Input: part model. Units: mm. Frame: model coordinates. A direction names the side the tool comes from. Coordinates: 2 decimals unless noted, no trailing zeros. Loops run counter-clockwise (first coordinate to the right, second up) from the corner with the lowest first, then second, coordinate; pieces in that order, holes last. Notation, with made-up numbers: (43, -40) - (71, -40) arc R22 cw to (71, -20) - close; hole circle Ø9 at (42.25, -2.75). An arc over 180 degrees is marked (long way). Write item = value, one per line. Start each with the question number.
from build123d import *

# Parameters (mm, degrees)
SERVO_ROD_HOLDERS_W                 = 10.16
SERVO_ROD_HOLDERS_H                 = 25.4
SERVO_ROD_HOLDERS_W_2               = 7.62
BASE_OF_THE_HOLDERS_DEPTH           = 0.508
SERVO_ROD_HOLDERS_3_W               = 7.62
SERVO_ROD_HOLDERS_3_H               = 25.4
TWO_HOLDERS_EXTRUDE_DEPTH           = 25.908
SKETCH2_R                           = 5.08
PLACEMENT_FOR_ROD_EXTRUDE_CUT_DEPTH = 25.4
SERVO_ROD_HOLDERS_4_W               = 12.7
SERVO_ROD_HOLDERS_4_H               = 25.4
EXTENSION_FOR_SCREWS_DEPTH          = 0.508


with BuildPart() as part:
    # Servo Rod Holders → Base of the Holders (new body)
    with BuildSketch(Plane.XY):
        with Locations((3.091913881, 0.940064131)):
            Rectangle(SERVO_ROD_HOLDERS_W, SERVO_ROD_HOLDERS_H)
        with Locations((-5.798086119, 0.940064131)):
            Rectangle(SERVO_ROD_HOLDERS_W_2, SERVO_ROD_HOLDERS_H)
        with Locations((11.981913881, 0.940064131)):
            Rectangle(SERVO_ROD_HOLDERS_W_2, SERVO_ROD_HOLDERS_H)
    extrude(amount=BASE_OF_THE_HOLDERS_DEPTH)

    # Servo Rod Holders_3 → Two Holders Extrude (add)
    with BuildSketch(Plane.XY):
        with Locations((11.981913881, 0.940064131)):
            Rectangle(SERVO_ROD_HOLDERS_3_W, SERVO_ROD_HOLDERS_3_H)
        with Locations((-5.798086119, 0.940064131)):
            Rectangle(SERVO_ROD_HOLDERS_3_W, SERVO_ROD_HOLDERS_3_H)
    extrude(amount=TWO_HOLDERS_EXTRUDE_DEPTH)

    # Sketch2 → Placement for Rod Extrude Cut (cut)
    with BuildSketch(Plane(origin=(15.791913881, 0, 0), x_dir=(0, 0, -1), z_dir=(1, 0, 0))):
        with Locations((-15.24, 0.940064131)):
            Circle(SKETCH2_R)
    extrude(amount=-PLACEMENT_FOR_ROD_EXTRUDE_CUT_DEPTH, mode=Mode.SUBTRACT)

    # Servo Rod Holders_4 → Extension for Screws (add)
    with BuildSketch(Plane.XY):
        with Locations((-15.958086119, 0.940064131)):
            Rectangle(SERVO_ROD_HOLDERS_4_W, SERVO_ROD_HOLDERS_4_H)
        with Locations((22.141913881, 0.940064131)):
            Rectangle(SERVO_ROD_HOLDERS_4_W, SERVO_ROD_HOLDERS_4_H)
    extrude(amount=EXTENSION_FOR_SCREWS_DEPTH)


solid = part.part
Item 1: Cut plane D-D on y = -2.5. Return loops of the section in (x, z), plus the area to 3 significant figures.
Item 2: Access query for faces 1 (the flat face through (-3, 13.64, 13)), 2 (the flat face through (22, 1, 0.508)), 3 (the flat face through (3, 1, 0.508)). Directions: +Z, -Z, +X, -X, +Y, -Y. A direction counts if a zero-diameter tool reaches every point of the face in a straight line with its end or side. Return the directions, or none.
Item 3: Pin query (flat end, axial travel): pin 1 (1.5 mm diameter, centred on y = 0, z = 22.5, fed in from -X); pin 2 (2 mm diameter, centred on y = 4, z = 23.5, fed in from +X); pin 3 (6.5 mm diameter, centred on x = 23.5, y = 1, fed in from +Z). Return the tip coordinate at first contact, or that it passes through.
Item 4: Cut plane A-A on z = 3. Return loops of the section in (x, y).
Item 5: Pull-direction query (Z, two-part tool) for faces 4 (the flat face through (-9.608, -2, 10)), 5 (the cylindrical face through (12.035, 2.466, 10.395)), 6 (the cylindrical face through (-5.745, 2.466, 10.395)), 7 (the flat face through (-16, 1, 0.508)); classes: pulls with the +Z half, pulls with the -Z half, needs draft (parallel to the pull), parting line crosses it, or undercut.
Item 6: Cut plane C-C on y = 7.25. Return loops of the section in (x, z), plus the area to 3 significant figures.
Item 7: Cut plane B-B on z = 15.24. Return loops of the section in (x, y).
Item 8: Ray query, line 1 (X direction, y = -7.25, z = 21); line 2 (Z direction, x = -14, y = -4.5); line 3 (Y direction, x = -5.75, z = 15.24). Return the intervals inside material, ascending.
Recorded:
q1.outline = (-22.31, 0) - (28.49, 0) - (28.49, 0.51) - (15.79, 0.51) - (15.79, 11.5) - (8.17, 11.5) - (8.17, 0.51) - (-1.99, 0.51) - (-1.99, 11.5) - (-9.61, 11.5) - (-9.61, 0.51) - (-22.31, 0.51) - close; (-9.61, 18.98) - (-1.99, 18.98) - (-1.99, 25.91) - (-9.61, 25.91) - close; (8.17, 18.98) - (15.79, 18.98) - (15.79, 25.91) - (8.17, 25.91) - close
q1.area = 299 mm²
q2.face_1 = +Z, -Z, +X, -X, +Y
q2.face_2 = +Z, +X, +Y, -Y
q2.face_3 = +Z, +Y, -Y
q3.pin_1 = -9.61
q3.pin_2 = 15.79
q3.pin_3 = 0.51
q4.outline = (-9.61, -11.76) - (-1.99, -11.76) - (-1.99, 13.64) - (-9.61, 13.64) - close; (8.17, -11.76) - (15.79, -11.76) - (15.79, 13.64) - (8.17, 13.64) - close
q5.face_4 = needs draft
q5.face_5 = undercut
q5.face_6 = undercut
q5.face_7 = pulls with the +Z half
q6.outline = (-22.31, 0) - (28.49, 0) - (28.49, 0.51) - (15.79, 0.51) - (15.79, 25.91) - (8.17, 25.91) - (8.17, 0.51) - (-1.99, 0.51) - (-1.99, 25.91) - (-9.61, 25.91) - (-9.61, 0.51) - (-22.31, 0.51) - close
q6.area = 413 mm²
q7.outline = (-9.61, -11.76) - (-1.99, -11.76) - (-1.99, -4.14) - (-9.61, -4.14) - close; (-9.61, 6.02) - (-1.99, 6.02) - (-1.99, 13.64) - (-9.61, 13.64) - close; (8.17, -11.76) - (15.79, -11.76) - (15.79, -4.14) - (8.17, -4.14) - close; (8.17, 6.02) - (15.79, 6.02) - (15.79, 13.64) - (8.17, 13.64) - close
q8.line_1 = -9.61 to -1.99, 8.17 to 15.79
q8.line_2 = 0 to 0.51
q8.line_3 = -11.76 to -4.14, 6.02 to 13.64
